Geometry: final body of the model. Coordinates: model frame, mm. A direction names the side the tool comes from. Give positions to 0.01 mm unless a question says otherwise; leave off trailing zeros. Write each loop counter-clockwise with the first axis right and the second up, starting at its lowest first coordinate (ties: lowest second). Pieces come first, ordered by that corner, then holes. Notation, with made-up numbers: M -1,-24 L 52,-24 A31 cw 52,8 Z; hole C -12.5,37.5 d10. An arc over 180 degrees is marked long. Use a Markdown table: item, result. Add a question column.
1) Section B-B on z = 3.85. State how many separate pieces and enclosed holes the cut face has, then the cut area to 3 significant figures.
2) Section D-D on y = -169.5. Return the cut outline in (x, z), then the cut area to 3 significant figures.
3) Draft query along X for faces 4 (the flat face through (-23.44, -177.7, 2.5)), 5 (the cylindrical face through (-41.179, -175.007, 2.504)), 6 (the cylindrical face through (-5.7, -160.1, 2.5)). Return one class per face: +X half, -X half, draft (parallel to the pull), parting line (faces both ways), or undercut.
4) Pin query (flat end, axial travel): pin 1 (2 mm diameter, centred on y = -179, z = 1, fed in from -X); pin 2 (3 mm diameter, centred on x = -3.5, z = 2.5, fed in from -Y). Return the tip coordinate at first contact, or that it passes through.
5) Section A-A on y = -177.8. Return the cut outline in (x, z), then the cut area to 3 significant figures.
6) Section C-C on x = -18. Return the cut outline in (y, z), then the cut area to 3 significant figures.
7) Set-up query: faces 1 (the flat face through (-5.575, -156, 3)), 2 (the cylindrical face through (5.816, -168.961, 2.504)), 3 (the flat face through (-45.159, -173.314, 2.504)). Return all of +Z, -Z, +X, -X, +Y, -Y with unobstructed straight access to the full face (end or side cutting, diameter ignored); none if empty.
8) Line query: line 1 (X direction, y = -152.4, z = 2.9); line 2 (X direction, y = -165.1, z = 1.7); line 3 (Y direction, x = 2, z = 0.4). Output: solid intervals per line, ascending.
Autodesk Inventor part; units mm, degrees
ref_plane "YZ Plane" through (0, 0, 0) normal (1, 0, 0) x (0, 1, 0)
ref_plane "XZ Plane" through (0, 0, 0) normal (0, 1, 0) x (-1, 0, 0)
ref_plane "XY Plane" through (0, 0, 0) normal (0, 0, 1) x (1, 0, 0)
sketch "Sketch2" plane through (0, 0, 0) normal (0, 0, 1) x (1, 0, 0)
  circle A0 centre (-50.0249, -177.8) radius 2.1844
  circle A1 centre (0.7751, -165.1) radius 2.1844
  circle A2 centre (0.7751, -152.4) radius 2.1844
  circle A3 centre (-50.0249, -152.4) radius 2.1844
  circle A4 centre (0.7751, -165.1) radius 6.35
  circle A5 centre (0.7751, -152.4) radius 6.35
  circle A6 centre (-50.0249, -177.8) radius 6.35
  line L0 (-5.5749, -131.829) -> (-5.5749, -160.1421)
  line L1 (-5.5749, -160.1421) -> (-51.565, -171.6396)
  line L2 (-50.6267, -184.4959) -> (7.1251, -170.0579)
  line L3 (7.1251, -170.0579) -> (7.1251, -148.3402)
  line L4 (-35.2436, -141.802) -> (-32.4116, -141.802)
  line L5 (-29.119, -141.802) -> (-26.287, -141.802)
  spline S0 degree 2 poles (-32.1725, -141.802) (-30.7653, -141.3711) (-29.3581, -141.802) knots 0 0 0 1 1 1 weights 1 1.034831 1
  spline S1 degree 3 poles (-18.0653, -168.2172) (-18.4536, -168.2172) (-18.8762, -168.1704) (-19.697, -167.9732) (-20.0954, -167.8231) (-20.8527, -167.4498) (-21.2719, -167.1795) (-22.0369, -166.5475) (-22.3831, -166.1864) (-22.9733, -165.4543) (-23.2675, -165.0121) (-23.7675, -164.0794) (-23.9738, -163.5891) (-24.3066, -162.6061) (-24.4533, -162.017) (-24.6377, -160.8215) (-24.6757, -160.2153) (-24.6621, -159.1128) (-24.6099, -158.5123) (-24.3986, -157.3309) (-24.2392, -156.75) (-23.8884, -155.7901) (-23.676, -155.3161) (-23.1679, -154.4164) (-22.8717, -153.9909) (-22.2831, -153.29) (-21.9408, -152.9459) (-21.1885, -152.3448) (-20.778, -152.0883) (-20.039, -151.7346) (-19.651, -151.5925) (-18.8526, -151.4059) (-18.4422, -151.3617) (-17.7112, -151.3617) (-17.3252, -151.4007) (-16.572, -151.5661) (-16.2047, -151.6923) (-15.5081, -152.0046) (-15.1205, -152.2298) (-14.403, -152.7599) (-14.0727, -153.0644) (-13.4595, -153.7287) (-13.1325, -154.1611) (-12.571, -155.0834) (-12.3359, -155.573) (-11.9434, -156.5769) (-11.7643, -157.1906) (-11.5273, -158.4416) (-11.469, -159.0789) (-11.4545, -160.2496) (-11.4978, -160.8932) (-11.7067, -162.1597) (-11.8725, -162.7825) (-12.2466, -163.8115) (-12.4761, -164.3187) (-13.0308, -165.2763) (-13.3566, -165.7263) (-13.9735, -166.4214) (-14.3085, -166.7415) (-15.0395, -167.2999) (-15.436, -167.5376) (-16.1507, -167.8676) (-16.528, -168.0009) (-17.3028, -168.1759) (-17.7004, -168.2172) (-18.0653, -168.2172) knots 0 0 0 0 0.1165 0.1165 0.232999 0.232999 0.369785 0.369785 0.506571 0.506571 0.651905 0.651905 0.797238 0.797238 0.963262 0.963262 1.129286 1.129286 1.294016 1.294016 1.458745 1.458745 1.600629 1.600629 1.742513 1.742513 1.875203 1.875203 2.007893 2.007893 2.120972 2.120972 2.234051 2.234051 2.340282 2.340282 2.446513 2.446513 2.569309 2.569309 2.692105 2.692105 2.84053 2.84053 2.988954 2.988954 3.163874 3.163874 3.338794 3.338794 3.515132 3.515132 3.69147 3.69147 3.843605 3.843605 3.99574 3.99574 4.122409 4.122409 4.249078 4.249078 4.358558 4.358558 4.468037 4.468037 4.468037 4.468037
  ellipse E0 centre (-18.0653, -159.6619) end of major axis (-18.0653, -154.3017) minor radius 4
  ellipse E1 centre (-18.0653, -159.6619) end of major axis (-18.0653, -161.1359) minor radius 1.1
  ellipse E2 centre (-18.0653, -127.6068) end of major axis (-18.0653, -163.5416) minor radius 12.1199 (-21.7061, -161.8819) -> (-21.3672, -162.1823) ccw
  ellipse E3 centre (-18.0653, -159.6619) end of major axis (-18.0653, -154.3017) minor radius 4 (-22.0428, -160.2294) -> (-21.7061, -161.8819) ccw
  ellipse E4 centre (-18.0653, -180.8584) end of major axis (-18.0653, -204.6203) minor radius 8.0143 (-21.8601, -159.929) -> (-22.0428, -160.2294) ccw
  line L6 (-21.8601, -159.929) -> (-20.5574, -159.929)
  ellipse E5 centre (-18.0653, -159.6619) end of major axis (-18.0653, -163.012) minor radius 2.5 (-15.5733, -159.929) -> (-20.5574, -159.929) ccw
  line L7 (-15.5733, -159.929) -> (-14.2705, -159.929)
  ellipse E6 centre (-18.0653, -180.8584) end of major axis (-18.0653, -204.6203) minor radius 8.0143 (-14.0878, -160.2294) -> (-14.2705, -159.929) ccw
  ellipse E7 centre (-18.0653, -159.6619) end of major axis (-18.0653, -154.3017) minor radius 4 (-14.4245, -161.8819) -> (-14.0878, -160.2294) ccw
  ellipse E8 centre (-18.0653, -127.6068) end of major axis (-18.0653, -163.5416) minor radius 12.1199 (-14.7634, -162.1823) -> (-14.4245, -161.8819) ccw
  line L8 (-14.7634, -162.1823) -> (-16.4184, -162.1823)
  ellipse E9 centre (-18.0653, -159.6619) end of major axis (-18.0653, -163.012) minor radius 2.5 (-19.7122, -162.1823) -> (-16.4184, -162.1823) ccw
  line L9 (-19.7122, -162.1823) -> (-21.3672, -162.1823)
  ellipse E10 centre (-18.0653, -159.6619) end of major axis (-18.0653, -158.3218) minor radius 1
  line L10 (-41.3127, -175.622) -> (-8.3483, -167.3809)
  line L11 (-8.3483, -167.3809) -> (-5.5749, -160.1421)
  line L12 (-41.3127, -175.622) -> (-49.0132, -171.0017)
  point P0 (0, 0)
  point P1 (-48.4848, -183.9604)
  point P2 (2.3152, -171.2604)
  point P3 (7.1251, -165.1)
  point P4 (7.1251, -152.4)
  point P5 (-5.5749, -152.4)
  dimension "d6" = 12.7
  dimension "d9" = 135
  dimension "d10" = 125
extrude "Extrusion2" add sketch "Sketch2" along normal blind 5.08 contours A4 | A4 A5 L3 | A4 L2 A6 L12 L10 L11 L0 A5 | A5 | A6 | L1 L12 A6
fillet "Fillet1" radius 7.62 4 edges at (-49.0132, -171.0017, 2.54) (-41.3127, -175.622, 2.54) (-8.3483, -167.3809, 2.54) (-5.5749, -160.1421, 2.54)
properties part number "back_funnel"
Found:
| question | item | result |
|---|---|---|
| 1 | separate pieces | 1 |
| 1 | enclosed holes | 3 |
| 1 | area | 656 mm² |
| 2 | outline | M -16.82,0 L 5.35,0 L 5.35,5.08 L -16.82,5.08 Z |
| 2 | area | 113 mm² |
| 3 | face 4 | +X half |
| 3 | face 5 | undercut |
| 3 | face 6 | -X half |
| 4 | pin 1 | x = -56.37 |
| 4 | pin 2 | y = -173.09 |
| 5 | outline | M -56.37,0 L -52.21,0 L -52.21,5.08 L -56.37,5.08 Z; M -47.84,0 L -23.84,0 L -23.84,5.08 L -47.84,5.08 Z |
| 5 | area | 143 mm² |
| 6 | outline | M -176.34,0 L -169.79,0 L -169.79,5.08 L -176.34,5.08 Z |
| 6 | area | 33.3 mm² |
| 7 | face 1 | +Z, -Z, -X, +Y |
| 7 | face 2 | +Z, -Z, +X, -Y |
| 7 | face 3 | +Z, -Z, +Y |
| 8 | line 1 | -5.57 to -1.41, 2.96 to 7.13 |
| 8 | line 2 | -7.65 to -1.41, 2.96 to 7.13 |
| 8 | line 3 | -171.34 to -166.91, -163.29 to -154.21, -150.59 to -146.17 |
